Study the drawing (mm; zero at the part's minimum x, y, z) and answer. A direction names the side the tool comes from. Coordinates: 2 decimals unless noted, no trailing zeros. Order: outer loops, then holes, each group sorted by start corner. A loop starts at its lowest first (then second) coordinate and runs counter-clockwise, first axis right, second up. Notation, with made-up numbers: M -17,47.25 L 6,47.25 A20 ccw 6,62.25 Z; hole C -21,86 d3. An arc over 180 degrees is marked long. Use a Markdown table: item, result. Add a question column.
1) Find section D-D on z = 2. Write down the section's boundary in (x, y).
2) Find section B-B on z = 9. Write down the section's boundary in (x, y), plus the area to 3 significant figures.
3) This flat-tipped pin is pushed along its axis until it touches: pin 1 Ø5 at (x, z) = (7, 8) entering from +Y. Where does it stop, or does it pass through?
4) The mould has two halves that part along Z. Classify the marked faces 3, 4 and 5: released by +Z, released by -Z, zero draft, split by the parting line, or undercut.
5) Find the intervals of material crossed by probe 1 along X at (y, z) = (16, 0.75); probe 2 along Z at (x, y) = (20.25, 12); probe 3 along Y at (x, z) = (25.3, 16.2), in increasing order. Write a range as [from, to].
6) For the marked faces 1 and 2, determine the directions among +Z, -Z, +X, -X, +Y, -Y from which every point of the face is accessible in a straight line to the end or side of a thin tool.
7) Find section A-A on y = 16. Write down the section's boundary in (x, z).
8) Find section C-C on y = 18.75. Write down the section's boundary in (x, z).
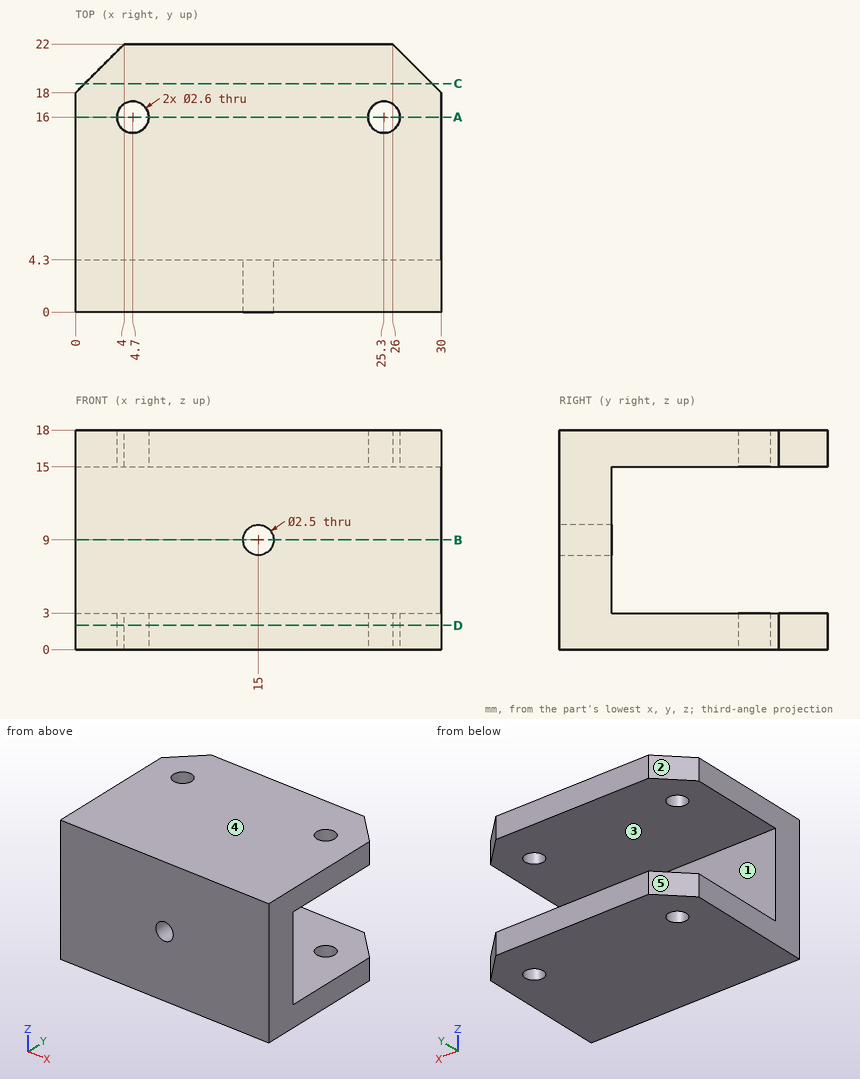
Check result:
| question | item | result |
|---|---|---|
| 1 | outline | M 0,0 L 30,0 L 30,18 L 26,22 L 4,22 L 0,18 Z; hole C 4.7,16 d2.6; hole C 25.3,16 d2.6 |
| 2 | outline | M 0,0 L 13.75,0 L 13.75,4.3 L 0,4.3 Z; M 16.25,0 L 30,0 L 30,4.3 L 16.25,4.3 Z |
| 2 | area | 118 mm2 |
| 3 | pin 1 | stops at y = 4.3 |
| 4 | face 3 | undercut |
| 4 | face 4 | released by +Z |
| 4 | face 5 | zero draft |
| 5 | probe 1 | x = [0, 3.4], [6, 24], [26.6, 30] |
| 5 | probe 2 | z = [0, 3], [15, 18] |
| 5 | probe 3 | y = [0, 14.7], [17.3, 22] |
| 6 | face 1 | +X, -X, +Y |
| 6 | face 2 | +Z, -Z, -X, +Y |
| 7 | outline | M 0,0 L 3.4,0 L 3.4,3 L 0,3 Z; M 0,15 L 3.4,15 L 3.4,18 L 0,18 Z; M 6,0 L 24,0 L 24,3 L 6,3 Z; M 6,15 L 24,15 L 24,18 L 6,18 Z; M 26.6,0 L 30,0 L 30,3 L 26.6,3 Z; M 26.6,15 L 30,15 L 30,18 L 26.6,18 Z |
| 8 | outline | M 0.75,0 L 29.25,0 L 29.25,3 L 0.75,3 Z; M 0.75,15 L 29.25,15 L 29.25,18 L 0.75,18 Z |
